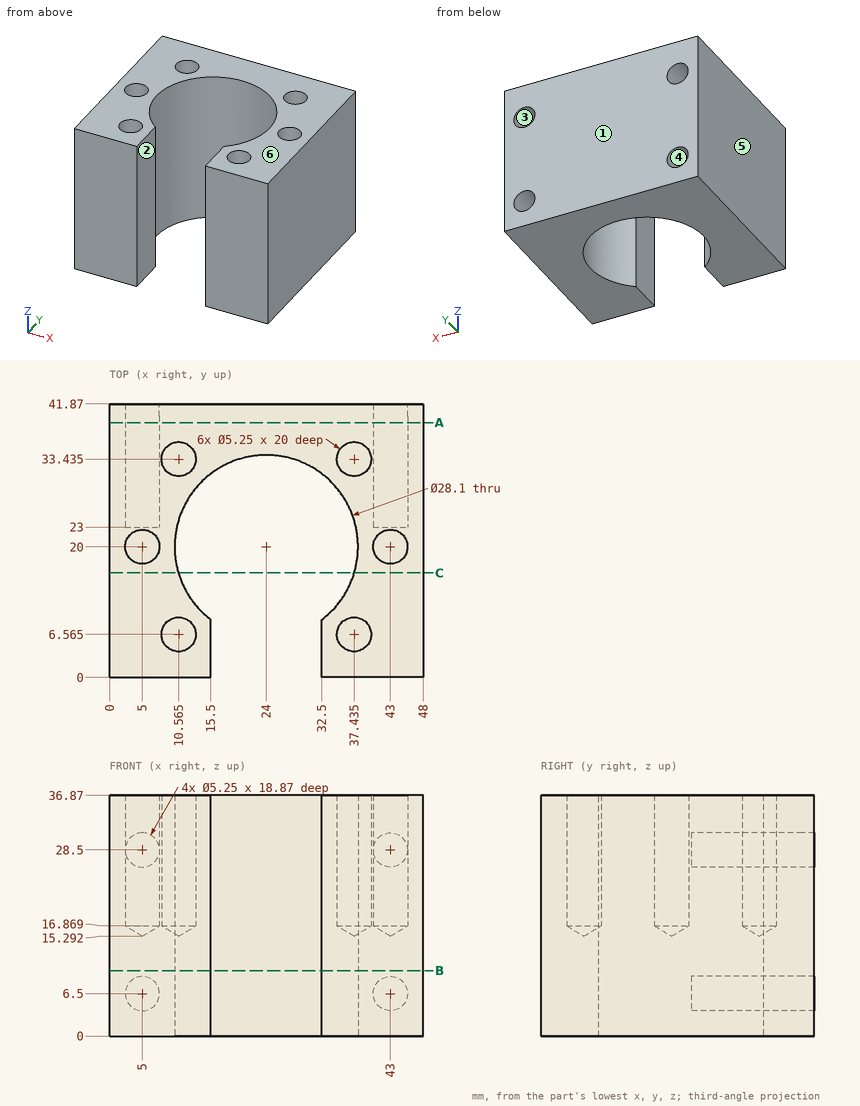
Can you work these out from the drawing? Everything is in mm from the part's minimum corner. A direction names the side the tool comes from. Give positions to 0.01 mm unless a question says otherwise; leave off trailing zeros. Loops run counter-clockwise (first coordinate to the right, second up) from the corner with the lowest first, then second, coordinate; pieces in that order, holes last. Notation, with made-up numbers: M 50.25,32 L 67.25,32 A24 cw 67.25,46 Z; hole C 49,37.5 d6. An arc over 180 degrees is marked long. Use CSV: the item, a comma, the result in double quotes. Start each with the question number.
1. If I drill on L1, parallel to X at y = 36.25, z = 6.5 (1 decimal); L2, parallel to Z at x = 5, y = 37.5 (1 decimal); L3, parallel to Y at x = 5, z = 25 (1 decimal), over which ranges is the centre line in solid material (lowest first)?
2. For P1, Ø4, axis at x = 5, z = 6.5, coming from the +Y side, with a flat end and sliding along its axis, tell me the tip position at first contact or that it passes through.
3. If we mould it in two halves opening along Z, with no side actions, what happens to the marked faces 4, 5 and 6? For each: released by +Z, released by -Z, zero draft, split by the parting line, or undercut.
4. On a 3-axis mill with a long thin cutter (end or side, diameter ignored), from which of +Z, -Z, +X, -X, +Y, -Y can I reach the whole of each face in a straight line? I mean the marked faces 1, 2 and 3. Say none if no direction works.
5. Imagine slicing it at C-C, the plane y = 16. Write out the boundary of the cut face in (x, z).
6. Imagine slicing it at A-A, the plane y = 39. Count the separate pieces of the cut face and the enclosed holes in it, plus the area to 3 significant figures.
7. Imagine slicing it at B-B, the plane z = 10. Write out the boundary of the cut face in (x, y).
Response values:
1,L1,"0 to 2.4, 7.6 to 40.4, 45.6 to 48"
1,L2,"0 to 3.9, 9.1 to 25.9, 31.1 to 36.9"
1,L3,"0 to 17.4, 22.6 to 41.9"
2,P1,"y = 23"
3,face 4,"undercut"
3,face 5,"zero draft"
3,face 6,"released by +Z"
4,face 1,"+Z, -Z, +X, -X, +Y"
4,face 2,"+Z, -Z, -Y"
4,face 3,"+Y"
5,outline,"M 0,0 L 10.53,0 L 10.53,36.87 L 0,36.87 Z; M 37.47,0 L 48,0 L 48,36.87 L 37.47,36.87 Z"
6,separate pieces,"1"
6,enclosed holes,"4"
6,area,"1,680 mm^2"
7,outline,"M 0,0 L 15.5,0 L 15.5,8.81 A14.05 cw long 32.5,8.81 L 32.5,0 L 48,0 L 48,41.87 L 0,41.87 Z"
